Print and shaded views of the part. All mm, measured from the part's lowest x, y and z. A direction names the side the tool comes from. Give positions to 0.01 mm unless a question says otherwise; leave off trailing zeros. Loops run counter-clockwise (first coordinate to the right, second up) from the corner with the lowest first, then second, coordinate; pieces in that order, holes last. Notation, with made-up numbers: M -32.5,-0.5 L 25.5,-0.5 A30 ccw 25.5,33.5 Z; hole C 88,48.5 d8. An arc over 180 degrees is marked long. Answer in a Markdown table with one row per item.
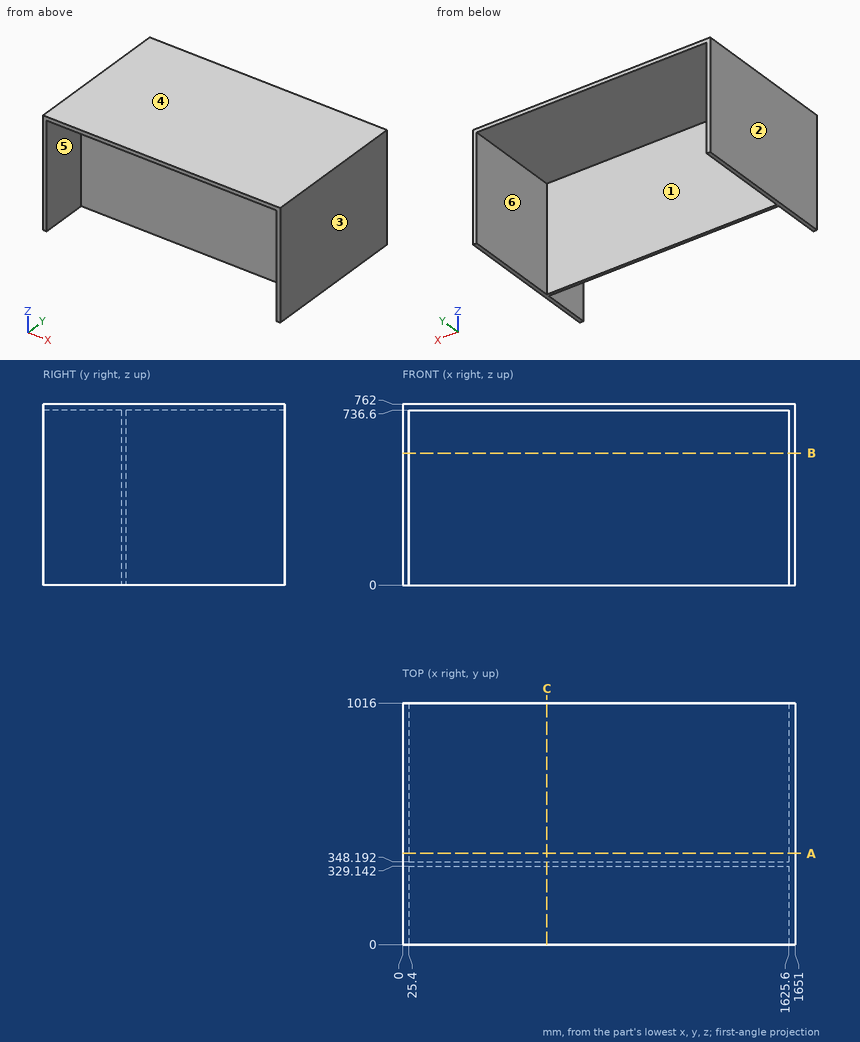
(1) Flat gauge pins, fed straight in: P1, Ø1.5, axis at x = 1303.5, y = 671.5, coming from the -Z side; P2, Ø5, axis at x = 988.5, z = 310.5, coming from the +Y side. Where does each tip first touch, or does it go through?
Established:
| item | result |
|---|---|
| P1 | stops at z = 736.6 |
| P2 | stops at y = 348.19 |
(2) Saw through at B-B, the plane z = 555.5. Give the cut face in (x, y), and give its area (3 significant figures).
Established:
| item | result |
|---|---|
| outline | M 0,0 L 25.4,0 L 25.4,329.14 L 1625.6,329.14 L 1625.6,0 L 1651,0 L 1651,1016 L 1625.6,1016 L 1625.6,348.19 L 25.4,348.19 L 25.4,1016 L 0,1016 Z |
| area | 82,100 mm2 |
(3) Mould opens along X. For the marked faces 1, 2 and 3 say: pulls with the +X half, pulls with the -X half, needs draft (parallel to the pull), parting line crosses it, or undercut.
Established:
| item | result |
|---|---|
| face 1 | undercut |
| face 2 | pulls with the -X half |
| face 3 | pulls with the +X half |
(4) Which spindle directions (+Z, -Z, +X, -X, +Y, -Y) get a long thin tool onto all of the face, cutting with end or side? Do the marked faces 4, 5 and 6. Say none if no direction does.
Established:
| item | result |
|---|---|
| face 4 | +Z, +X, -X, +Y, -Y |
| face 5 | -Z, -Y |
| face 6 | -Z, +Y |
(5) Saw through at A-A, the plane y = 384.5. Give the cut face in (x, z).
Established:
| item | result |
|---|---|
| outline | M 0,0 L 25.4,0 L 25.4,736.6 L 1625.6,736.6 L 1625.6,0 L 1651,0 L 1651,762 L 0,762 Z |
(6) Saw through at C-C, the plane x = 607.5. Give the cut face in (y, z).
Established:
| item | result |
|---|---|
| outline | M 0,736.6 L 329.14,736.6 L 329.14,0 L 348.19,0 L 348.19,736.6 L 1016,736.6 L 1016,762 L 0,762 Z |
(7) Wall check: L1, parallel to X at y = 648, z = 521.5; L2, parallel to Y at x = 1030.5, z = 499.5; L3, parallel to Z at x = 325, y = 575.5. Give the ranges that are in metal, low to high.
Established:
| item | result |
|---|---|
| L1 | x = 0 to 25.4, 1625.6 to 1651 |
| L2 | y = 329.14 to 348.19 |
| L3 | z = 736.6 to 762 |
